Autodesk Inventor part; units mm, degrees
ref_plane "YZ Plane" through (0, 0, 0) normal (1, 0, 0) x (0, 1, 0)
ref_plane "XZ Plane" through (0, 0, 0) normal (0, 1, 0) x (-1, 0, 0)
ref_plane "XY Plane" through (0, 0, 0) normal (0, 0, 1) x (1, 0, 0)
sketch "Sketch1" plane through (0, 0, 0) normal (0, 0, 1) x (1, 0, 0)
  line L0 (24.1101, 25.4) -> (24.1101, 0)
  line L1 (24.1101, 0) -> (-20.3399, 0)
  line L2 (-20.3399, 0) -> (-20.3399, 25.4)
  line L3 (-17.1649, 25.4) -> (-17.1649, 3.175)
  line L4 (-17.1649, 3.175) -> (20.9351, 3.175)
  line L5 (20.9351, 3.175) -> (20.9351, 25.4)
  line L6 (-20.3399, 25.4) -> (-17.1649, 25.4)
  line L7 (24.1101, 25.4) -> (20.9351, 25.4)
  point P0 (0, 0)
  dimension "d0" = 44.45
  dimension "d1" = 25.4
  dimension "d2" = 3.175
extrude "Extrusion1" add sketch "Sketch1" against normal blind 152.4
sketch "Sketch5" plane through (-20.3399, 0, 0) normal (0, -1, 0) x (1, 0, 0)
  line L0 (0, 0) -> (44.45, 0)
  line L1 (44.45, 0) -> (44.45, -152.4)
  line L2 (44.45, -152.4) -> (44.45, -41.275)
  line L3 (44.45, 0) -> (44.45, -152.4)
  line L4 (44.45, -41.275) -> (12.2024, 0)
  line L5 (12.2024, 0) -> (44.45, 0)
  line L6 (44.45, 0) -> (44.45, -41.275)
  point P0 (20.3399, 0)
  dimension "d14" = 111.125
  dimension "d15" = 38
extrude "Extrusion4" cut sketch "Sketch5" against normal through all
properties part number "Horizontal channel right"
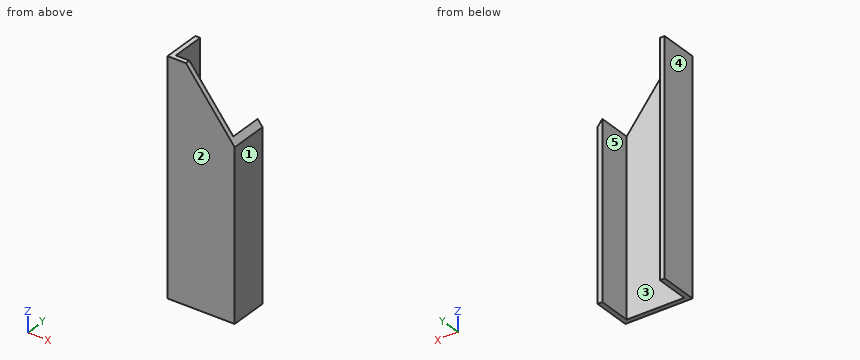
Input: part model. Units: mm. Frame: model coordinates. Face numbers are marked on the shaded views. A direction names the side the tool comes from. Give positions to 0.01 mm unless a question says otherwise; leave off trailing zeros. Order: outer loops, then holes, each group sorted by start corner. A loop starts at its lowest first (then second) coordinate and runs counter-clockwise, first axis right, second up. Notation, with made-up numbers: M 18,-4.5 L 52,-4.5 A17 ccw 52,0.5 Z; hole C 61,60 d9. An arc over 180 degrees is marked long. Answer as a JSON object with one key per item and string values.
1. Cut plane A-A, the plane y = 10. Output: boundary loops of the cut face in (x, z) (3 decimals).
Result sheet:
{"outline": "M -20.34,-152.4 L -17.165,-152.4 L -17.165,0 L -20.34,0 Z; M 20.935,-152.4 L 24.11,-152.4 L 24.11,-41.275 L 20.935,-37.211 Z"}
2. Reachability of the marked faces 4 and 5 from +Z, -Z, +X, -X, +Y, -Y: full face, straight path, thin tool, end or side. Return the list, or none.
Result sheet:
{"face 4": "+Z, -Z, -X, +Y, -Y", "face 5": "+Z, -Z, +Y"}
3. Ray query, line 1 (X direction, y = 14.5, z = -70.5); line 2 (Y direction, x = 4, z = -114.5) (3 decimals); line 3 (X direction, y = 7.25, z = -13). Return the intervals inside material, ascending. Write a range as [from, to].
Result sheet:
{"line 1": "[-20.34, -17.16], [20.94, 24.11]", "line 2": "[0, 3.175]", "line 3": "[-20.34, -17.16]"}
4. Cut plane D-D, the plane z = -14.5. Output: boundary loops of the cut face in (x, y) (3 decimals).
Result sheet:
{"outline": "M -20.34,0 L 3.191,0 L 3.191,3.175 L -17.165,3.175 L -17.165,25.4 L -20.34,25.4 Z"}
5. Cut plane C-C, the plane x = 14. Output: boundary loops of the cut face in (y, z) (3 decimals).
Result sheet:
{"outline": "M 0,-152.4 L 3.175,-152.4 L 3.175,-28.335 L 0,-28.335 Z"}
6. Pull-direction query (X, two-part tool) for the marked faces 1, 2 and 3; classes: +X half, -X half, draft (parallel to the pull), parting line (faces both ways), or undercut.
Result sheet:
{"face 1": "+X half", "face 2": "draft", "face 3": "undercut"}
7. Cut plane B-B, the plane z = -63. Output: boundary loops of the cut face in (x, y) (3 decimals), and give its area (3 significant figures).
Result sheet:
{"outline": "M -20.34,0 L 24.11,0 L 24.11,25.4 L 20.935,25.4 L 20.935,3.175 L -17.165,3.175 L -17.165,25.4 L -20.34,25.4 Z", "area": "282 mm²"}
